Can you work these out from the model? Positions are in its coordinate system, mm. A direction names the side the tool comes from. Coordinates: 2 decimals unless noted, no trailing zeros. Order: outer loops, then holes, each group sorted by start corner. A loop starts at its lowest first (then second) coordinate and runs counter-clockwise, first axis right, second up. Notation, with made-up numbers: (12.25, 16) -> (60.25, 16) arc R21 cw to (60.25, 21) -> close; hole circle Ø6 at (-16.75, 39). An arc over 180 degrees is marked (long way). Answer in a Markdown table with one row per item.
```python
from build123d import *

# Parameters (mm, degrees)
SKETCH1_R           = 2.5
BOSS_EXTRUDE2_DEPTH = 14.72
CUT_SWEEP1_START    = 8.3
CUT_SWEEP1_DEPTH    = 1.47


# Read off the part's stored shape, not the designer's step: Cut-Sweep1
with BuildPart() as part:
    # Sketch1 → Boss-Extrude2 (new body)
    with BuildSketch(Plane(origin=(0, 0, 0), x_dir=(1, 0, 0), z_dir=(0, 1, 0))):
        with BuildLine():
            Line((-12.15, -5), (12.15, -5))
            ThreePointArc((12.15, -5), (13.564213562, -4.414213562), (14.15, -3))
            Line((14.15, -3), (14.15, 3))
            ThreePointArc((14.15, 3), (13.564213562, 4.414213562), (12.15, 5))
            Line((12.15, 5), (4.92, 5))
            Line((4.92, 5), (3.58, 3.75))
            Line((3.58, 3.75), (-3.58, 3.75))
            Line((-3.58, 3.75), (-4.92, 5))
            Line((-4.92, 5), (-12.15, 5))
            ThreePointArc((-12.15, 5), (-13.564213562, 4.414213562), (-14.15, 3))
            Line((-14.15, 3), (-14.15, -3))
            ThreePointArc((-14.15, -3), (-13.564213562, -4.414213562), (-12.15, -5))
        make_face()
        with Locations(Location((7.85, 0, 0), (0, 0, 270))):
            Circle(SKETCH1_R, mode=Mode.SUBTRACT)
        with Locations(Location((-10.1, 0, 0), (0, 0, 270))):
            Circle(SKETCH1_R, mode=Mode.SUBTRACT)
        with BuildLine():
            Line((-2.631143176, 1.995377842), (-2.646508574, -1.983686381))
            ThreePointArc((-2.646508574, -1.983686381), (1.374981361, -0.00965383), (-2.631143176, 1.995377842))
        make_face(mode=Mode.SUBTRACT)
    extrude(amount=BOSS_EXTRUDE2_DEPTH)

    # Cut-Sweep1 outline → Cut-Sweep1 (cut)
    with BuildSketch(Plane(origin=(0, 0, 0), x_dir=(1, 0, 0), z_dir=(0, 1, 0)).offset(CUT_SWEEP1_START)):
        with BuildLine():
            ThreePointArc((-12.15, 5), (-13.564213562, 4.414213562), (-14.15, 3))
            Line((-14.15, 3), (-14.15, -3))
            ThreePointArc((-14.15, -3), (-13.564213562, -4.414213562), (-12.15, -5))
            Line((-12.15, -5), (12.15, -5))
            ThreePointArc((12.15, -5), (13.564213562, -4.414213562), (14.15, -3))
            Line((14.15, -3), (14.15, 3))
            ThreePointArc((14.15, 3), (13.564213562, 4.414213562), (12.15, 5))
            Line((12.15, 5), (4.92, 5))
            Line((4.92, 5), (3.58, 3.75))
            Line((3.58, 3.75), (-3.58, 3.75))
            Line((-3.58, 3.75), (-4.92, 5))
            Line((-4.92, 5), (-12.15, 5))
        make_face()
        with BuildLine():
            ThreePointArc((-12.22, -1.324990566), (-12.6, 0), (-12.22, 1.324990566))
            Line((-12.22, 1.324990566), (-12.22, 3))
            ThreePointArc((-12.22, 3), (-12.199497475, 3.049497475), (-12.15, 3.07))
            Line((-12.15, 3.07), (12.15, 3.07))
            ThreePointArc((12.15, 3.07), (12.199497475, 3.049497475), (12.22, 3))
            Line((12.22, 3), (12.22, -3))
            ThreePointArc((12.22, -3), (12.199497475, -3.049497475), (12.15, -3.07))
            Line((12.15, -3.07), (-12.15, -3.07))
            ThreePointArc((-12.15, -3.07), (-12.199497475, -3.049497475), (-12.22, -3))
            Line((-12.22, -3), (-12.22, -1.324990566))
        make_face(mode=Mode.SUBTRACT)
    extrude(amount=CUT_SWEEP1_DEPTH, mode=Mode.SUBTRACT)


solid = part.part
```
(1) Suppose I cut it at C-C (z = 0). Please give me the cut outline in (x, y) (3 decimals), and give its area (3 significant figures).
Response values:
| item | result |
|---|---|
| outline | (-14.15, 0) -> (-12.6, 0) -> (-12.6, 8.3) -> (-14.15, 8.3) -> close; (-14.15, 9.77) -> (-12.6, 9.77) -> (-12.6, 14.72) -> (-14.15, 14.72) -> close; (-7.6, 0) -> (-2.639, 0) -> (-2.639, 14.72) -> (-7.6, 14.72) -> close; (1.375, 0) -> (5.35, 0) -> (5.35, 14.72) -> (1.375, 14.72) -> close; (10.35, 0) -> (14.15, 0) -> (14.15, 8.3) -> (12.22, 8.3) -> (12.22, 9.77) -> (14.15, 9.77) -> (14.15, 14.72) -> (10.35, 14.72) -> close |
| area | 205 mm2 |
(2) Will these pins go through, and if not, where does the flat tip stop? pin 1 Ø1.2 at (x, y) = (-0.5, 9.5) entering from -Z; pin 2 Ø0.7 at (y, z) = (9, -2) entering from -X.
Response values:
| item | result |
|---|---|
| pin 1 | z = -3.75 |
| pin 2 | x = -12.22 |
(3) Suppose I cut it at A-A (x = -10.1). Please give me the cut outline in (y, z).
Response values:
| item | result |
|---|---|
| outline | (0, -5) -> (8.3, -5) -> (8.3, -3.07) -> (9.77, -3.07) -> (9.77, -5) -> (14.72, -5) -> (14.72, -2.5) -> (0, -2.5) -> close; (0, 2.5) -> (14.72, 2.5) -> (14.72, 5) -> (9.77, 5) -> (9.77, 3.07) -> (8.3, 3.07) -> (8.3, 5) -> (0, 5) -> close |
(4) We'd pull the mould along Z, two halves only. Please class faces 1 (the cylindrical face through (-13.58, 12.21, 4.4)), 2 (the cylindrical face through (10.33, 7.26, -0.33)), 3 (the flat face through (14.15, 12, 0)): +Z half, -Z half, draft (parallel to the pull), parting line (faces both ways), or undercut.
Response values:
| item | result |
|---|---|
| face 1 | +Z half |
| face 2 | undercut |
| face 3 | draft |
(5) I need wall thicknesses on line 1 (X direction, y = 6.25, z = 0) (3 decimals); line 2 (X direction, y = 8.5, z = 0) (3 decimals); line 3 (Y direction, x = 7.75, z = 3.5). Which ranges of each line are inside material? Lowest first, please. Write a range as [from, to].
Response values:
| item | result |
|---|---|
| line 1 | [-14.15, -12.6], [-7.6, -2.639], [1.375, 5.35], [10.35, 14.15] |
| line 2 | [-7.6, -2.639], [1.375, 5.35], [10.35, 12.22] |
| line 3 | [0, 8.3], [9.77, 14.72] |
(6) Suppose I cut it at B-B (y = 4). Count the separate pieces of the cut face and the enclosed holes in it, and give its area (3 significant figures).
Response values:
| item | result |
|---|---|
| separate pieces | 1 |
| enclosed holes | 3 |
| area | 213 mm2 |
(7) On a 3-axis mill with a long thin cutter (end or side, diameter ignored), from which of +Z, -Z, +X, -X, +Y, -Y can I reach the whole of each face in a straight line? I mean faces 4 (the flat face through (-4.241, 4.092, -4.366)), 5 (the flat face through (0, 9, 3.07)), 6 (the cylindrical face through (-13.55, 4.09, -4.43)). Say none if no direction works.
Response values:
| item | result |
|---|---|
| face 4 | -Z, +Y, -Y |
| face 5 | +Z, +X, -X |
| face 6 | -Z, -X, +Y, -Y |
(8) Suppose I cut it at D-D (x = -6). Please give me the cut outline in (y, z), and give its area (3 significant figures).
Response values:
| item | result |
|---|---|
| outline | (0, -5) -> (8.3, -5) -> (8.3, -3.07) -> (9.77, -3.07) -> (9.77, -5) -> (14.72, -5) -> (14.72, 5) -> (9.77, 5) -> (9.77, 3.07) -> (8.3, 3.07) -> (8.3, 5) -> (0, 5) -> close |
| area | 142 mm2 |
